Autodesk Inventor part; units mm, degrees
ref_plane "YZ Plane" through (0, 0, 0) normal (1, 0, 0) x (0, 1, 0)
ref_plane "XZ Plane" through (0, 0, 0) normal (0, 1, 0) x (-1, 0, 0)
ref_plane "XY Plane" through (0, 0, 0) normal (0, 0, 1) x (1, 0, 0)
sketch "Sketch1" plane through (0, 0, 0) normal (0, 0, 1) x (1, 0, 0)
  line L0 (0, 0) -> (0, 56.35)
  line L1 (0, 56.35) -> (26.1, 56.35)
  line L2 (26.1, 56.35) -> (26.1, 31.35)
  line L3 (26.1, 31.35) -> (19.75, 25)
  line L4 (19.75, 25) -> (19.75, 0)
  line L5 (19.75, 0) -> (0, 0)
  dimension "d1" = 39.5
  dimension "d3" = 45
  dimension "d5" = 52.2
  dimension "d6" = 25
revolve "Revolution1" add sketch "Sketch1" angle 360 about axis through (0, 0, 0) along (0, -1, 0)
fillet "Fillet2" radius 2 1 edges at (-19.75, 25, 0)
fillet "Fillet3" radius 2 1 edges at (-26.1, 31.35, 0)
shell "Shell2" thickness 2.5 removed faces 2 at (7.4507, 56.35, 1.961) at (5.8293, 0, 3.0594)
ref_plane "Work Plane4" through (-19.7215, 58.7231, 59.4617) normal (0, 1, 0) x (-0.9806, 0, 0.1963)
ref_plane "Work Plane2" through (-19.7215, 0.4561, 59.4617) normal (0, 1, 0) x (-0.9806, 0, 0.1963)
ref_plane "Work Plane5" through (-19.7215, 52.7231, 59.4617) normal (0, 1, 0) x (-0.9806, 0, 0.1963)
sketch "Sketch5" plane through (-19.7215, 52.7231, 59.4617) normal (0, 1, 0) x (-0.9806, 0, 0.1963)
  circle A0 centre (-31.0082, -54.4346) radius 26.1
  line L0 (-8, -28.3346) -> (-8, -14.4346)
  line L1 (-8, -14.4346) -> (0, -14.4346)
  line L2 (0, -14.4346) -> (0, -94.4346)
  line L3 (0, -94.4346) -> (-8, -94.4346)
  line L4 (0, 0) -> (0, -15)
  line L5 (-8, -94.4346) -> (-8, -80.5346)
  line L6 (-8, -80.5346) -> (-31.0082, -80.5346)
  line L7 (-31.0082, -28.3346) -> (-8, -28.3346)
  point P0 (-31.0082, -54.4346)
  dimension "d20" = 40
  dimension "d21" = 40
  dimension "d22" = 8
extrude "Extrusion2" add sketch "Sketch5" against normal blind 15 contours A0 L7 L0 L1 L2 L3 L5 L6
sketch "Sketch6" plane through (-27.6833, 37.7231, -21.0766) normal (0.9806, 0, -0.1963) x (-0.1963, 0, -0.9806)
  point P0 (-26.1, -37.7231)
ref_plane "Work Plane6" through (0, 43.85, 0) normal (-0.1963, 0, -0.9806) x (0, -1, 0)
sketch "Sketch7" plane through (-27.6833, 37.7231, -21.0766) normal (0.9806, 0, -0.1963) x (-0.1963, 0, -0.9806)
  line L0 (0, 15) -> (13.9, 15)
  line L1 (13.9, 15) -> (13.9, 0)
  point P0 (-26.1, -37.7231)
  point P1 (6.9, 7.5)
  dimension "d27" = 7.5
  dimension "d35" = 7
hole "Hole1" at (-29.0375, 45.2231, -27.8424) direction (-0.9806, 0, 0.1963) diameter 4.5 end through all
mirror "Mirror1" about plane through (0, 43.85, 0) normal (-0.1963, 0, -0.9806) of "Hole1"
chamfer "Chamfer2" distance 4 angle 45 2 edges at (-28.5959, 45.2231, -25.6362) (-16.5256, 45.2231, 34.6677)
properties part number "_3DPrint"
The listing builds one solid part. Answer for the finished solid, in the listing's coordinates (mm). A direction names the side the tool comes from. Coordinates: 2 decimals unless noted, no trailing zeros. Order: outer loops, then holes, each group sorted by start corner. A loop starts at its lowest first (then second) coordinate and runs counter-clockwise, first axis right, second up.
Q1. Consider line 1 (X direction, y = 18, z = 0); line 2 (Z direction, x = 0, y = 42). Determine where each line is inside the solid, lowest interval first.
Q2. Given P1, Ø4, axis at y = 40, z = -11.5, coming from the -X side; P2, Ø4, axis at y = 32.5, z = 3.5, coming from the +X side; P3, Ø12, axis at y = 7, z = 7.5, coming from the +X side; P4, Ø13, axis at x = -10.5, z = 12.5, coming from the -Y side, each flat-ended and moving along its own axis, determine where each tip first touches the part or whether it passes through.
Q3. Which of the six approach directions +Z, -Z, +X, -X, +Y, -Y give full straight-line access (tool end or side, diameter ignored) to faces 5 (the face through (-23.577, 44.2, 1.038)), 6 (the face through (12.044, 44.095, -23.155)), 7 (the face through (-16.563, 45.328, -23.303))?
Q4. A cutting plane is placed at B-B, the plane x = -16. State how many separate pieces and enclosed holes the cut face has, and give its area (3 significant figures).
Q5. A cutting plane is placed at A-A, the plane y = 4.5. Write down the section's boundary in (x, z).
Q6. For a pull along Y with two mould halves and no side action, classify faces 1 (the face through (-33.184, 45.974, -29.444)), 2 (the face through (10.151, 27.668, -15.922)), 3 (the face through (-34.85, 47.42, -26.18)), 4 (the face through (-14.6, 11.9, 13.3)) as pulls with the +Y half, pulls with the -Y half, needs draft (parallel to the pull), parting line crosses it, or undercut.
Answers follow:
1. line 1: x = -19.75 to -17.25, 17.25 to 19.75
1. line 2: z = -26.1 to -23.6, 23.6 to 26.62
2. P1: stops at x = -34.33
2. P2: stops at x = 26.06
2. P3: stops at x = 19.69
2. P4: stops at y = 0
3. face 5: +Y
3. face 6: none
3. face 7: -Z, +Y, -Y
4. separate pieces: 5
4. enclosed holes: 0
4. area: 725 mm2
5. outline: circle Ø39.5 at (0, 0); hole circle Ø34.5 at (0, 0)
6. face 1: undercut
6. face 2: pulls with the +Y half
6. face 3: undercut
6. face 4: needs draft
